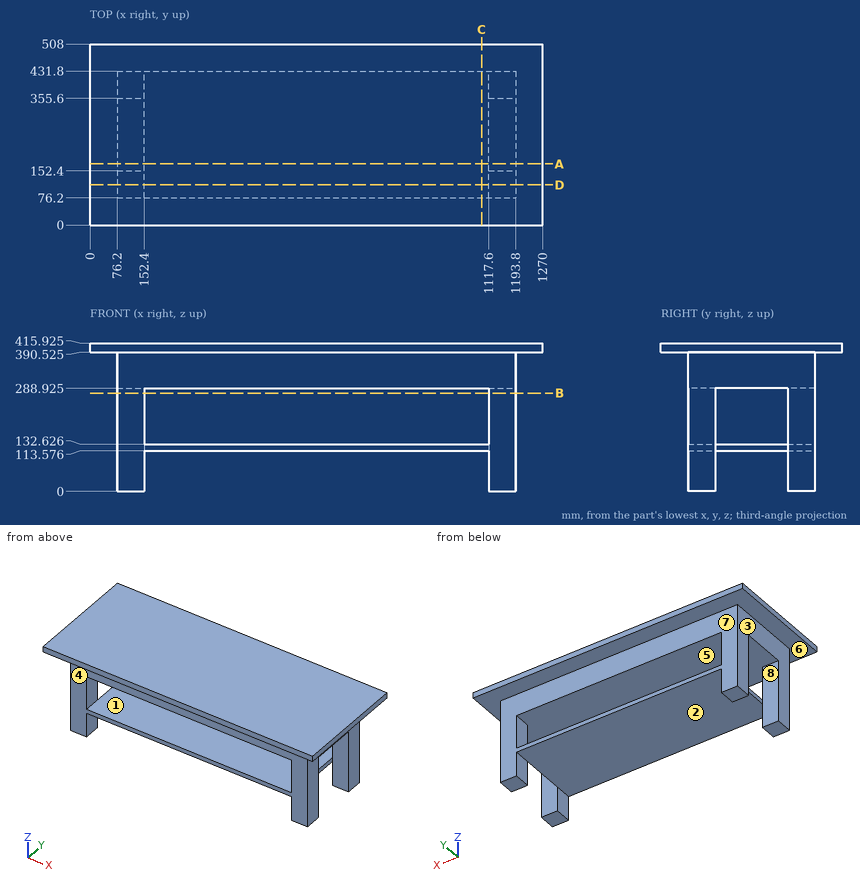
For this review, use the dimensioned drawing (mm, ordinates from the lowest corner) and the shaded views. A direction names the side the tool comes from. Give positions to 0.01 mm unless a question says otherwise; leave off trailing zeros. Write each loop counter-clockwise with the first axis right and the second up, starting at its lowest first coordinate (ties: lowest second). Pieces come first, ordered by that corner, then holes. Notation, with made-up numbers: M 38,47.25 L 82,47.25 A23 ccw 82,75.25 Z; hole C -37,-6 d6. An arc over 180 degrees is marked long. Answer as a JSON object with one key per item and string values. Group by question number.
1) For line 1 along Z through (x, y) = (923, 257) (3 decimals); line 2 along Z through (x, y) = (668, 480) (3 decimals); line 3 along Y through (x, z) = (98.5, 116), list the stretches that pass through material, from the lowest coordinate up.
2) Clearance check with flat-ended pins moving along their axes: pin 1 Ø3 at (y, z) = (232.5, 133) entering from +X; pin 2 Ø5 at (y, z) = (158, 337.5) entering from -X; pin 3 Ø23 at (y, z) = (395, 63) entering from +X. State where each tip first meets the part, or that it passes through.
3) We need section C-C (x = 1098.5). Give the boundary of the cut face in (y, z) (3 decimals).
4) We need section A-A (y = 171.5). Give the boundary of the cut face in (x, z) (3 decimals), and give its area (3 significant figures).
5) Mouldability with a two-part tool opening along Y and no side actions: class the marked faces 6, 7 and 8 as released by +Y, released by -Y, zero draft, split by the parting line, or undercut.
6) Tool access review of the marked faces 1, 2, 3, 4 and 5: name each direction out of +Z, -Z, +X, -X, +Y, -Y from which nothing blocks a thin tool from reaching the whole face with its end or side.
7) We need section D-D (y = 113). Give the boundary of the cut face in (x, z) (3 decimals).
8) We need section B-B (z = 276). Give the boundary of the cut face in (x, y).
Answer key:
{
 "1": {"line 1": "z = 113.576 to 132.626, 288.925 to 415.925", "line 2": "z = 390.525 to 415.925", "line 3": "y = 76.2 to 152.4, 355.6 to 431.8"},
 "2": {"pin 1": "stops at x = 1117.6", "pin 2": "stops at x = 76.2", "pin 3": "stops at x = 1193.8"},
 "3": {"outline": "M 0,390.525 L 76.2,390.525 L 76.2,288.925 L 431.8,288.925 L 431.8,390.525 L 508,390.525 L 508,415.925 L 0,415.925 Z; M 76.2,113.576 L 431.8,113.576 L 431.8,132.626 L 76.2,132.626 Z"},
 "4": {"outline": "M 0,390.525 L 76.2,390.525 L 76.2,288.925 L 1193.8,288.925 L 1193.8,390.525 L 1270,390.525 L 1270,415.925 L 0,415.925 Z; M 152.4,113.576 L 1117.6,113.576 L 1117.6,132.626 L 152.4,132.626 Z", "area": "164,000 mm²"},
 "5": {"face 6": "zero draft", "face 7": "released by +Y", "face 8": "undercut"},
 "6": {"face 1": "+Y, -Y", "face 2": "-Z, +Y, -Y", "face 3": "-Z, -X, +Y, -Y", "face 4": "-Z, +X, -X, -Y", "face 5": "none"},
 "7": {"outline": "M 0,390.525 L 76.2,390.525 L 76.2,0 L 152.4,0 L 152.4,113.576 L 1117.6,113.576 L 1117.6,0 L 1193.8,0 L 1193.8,390.525 L 1270,390.525 L 1270,415.925 L 0,415.925 Z; hole M 152.4,132.626 L 1117.6,132.626 L 1117.6,288.925 L 152.4,288.925 Z"},
 "8": {"outline": "M 76.2,76.2 L 152.4,76.2 L 152.4,152.4 L 76.2,152.4 Z; M 76.2,355.6 L 152.4,355.6 L 152.4,431.8 L 76.2,431.8 Z; M 1117.6,76.2 L 1193.8,76.2 L 1193.8,152.4 L 1117.6,152.4 Z; M 1117.6,355.6 L 1193.8,355.6 L 1193.8,431.8 L 1117.6,431.8 Z"}
}
